```python
from build123d import *

# Parameters (mm, degrees)
F0_R     = 15.875
F1_DEPTH = 5.08
F2_R     = 17.78
F3_DEPTH = 5.08
F4_R     = 9.525
F5_DEPTH = 3.302


with BuildPart() as f1:
    # F0 (on Right) → F1 (new body)
    with BuildSketch(Plane.YZ):
        Circle(F0_R)
        Polygon((0, -14.664697), (-12.7, -7.332348), (-12.7, 7.332348), (0, 14.664697), (12.7, 7.332348), (12.7, -7.332348), align=None, mode=Mode.SUBTRACT)
    extrude(amount=F1_DEPTH)

    # F2 (on face) → F3 (join)
    with BuildSketch(Plane.YZ.offset(5.08)):
        Circle(F2_R)
    extrude(amount=F3_DEPTH)

    # F4 (on face) → F5 (cut)
    with BuildSketch(Plane(origin=(5.08, 0, 0), x_dir=(0, -1, 0), z_dir=(-1, 0, 0))):
        Circle(F4_R)
    extrude(amount=-F5_DEPTH, mode=Mode.SUBTRACT)


solid = f1.part
```
Check sheet for the modelled part. Datum: model origin and axes. Units: mm. A direction names the side the tool comes from. Coordinates: 2 decimals unless noted, no trailing zeros. Write each loop counter-clockwise with the first axis right and the second up, starting at its lowest first coordinate (ties: lowest second). Pieces come first, ordered by that corner, then holes. Notation, with made-up numbers: M 10.25,73.5 L 53.25,73.5 A25 ccw 53.25,104.5 Z; hole C 50,10.25 d3. An arc over 180 degrees is marked long. Write item = value, one per line. Start each with the question number.
1. Sectioned sample at B-B (z = 0). Record the cut outline in (x, y) (3 decimals), then the cut area to 3 significant figures.
2. Thickness scan on probe 1 along Z at (x, y) = (6.65, 0) (3 decimals); probe 2 along X at (y, z) = (-5, 2.5); probe 3 along X at (y, z) = (8, 8). Record the ranges inside material, lowest first.
3. Go/stop test with flat-tipped pins: pin 1 (1.5 mm diameter, centred on x = 1.5, z = -2, fed in from +Y); pin 2 (15 mm diameter, centred on y = 3.5, z = -3.5, fed in from -X); pin 3 (2.5 mm diameter, centred on x = 2.5, z = -2, fed in from -Y). Record where each tip stops, or that it passes through.
4. Sectioned sample at C-C (y = -11). Record the cut outline in (x, z).
5. Sectioned sample at A-A (x = 4.5). Record the cut outline in (y, z) (3 decimals).
6. Mould release check, pull along Y, two halves, no side actions. Record for faces 1 (the cylindrical face through (6.708, 7.559, -5.796)), 2 (the flat face through (8.382, 0, 0)), 3 (the cylindrical face through (7.58, -3.85, -17.36)), 4 (the flat face through (0, 7, 11)): pulls with the +Y half, pulls with the -Y half, needs draft (parallel to the pull), parting line crosses it, or undercut.
7. Sectioned sample at D-D (y = -4.5). Record the cut outline in (x, z).
8. Tool access check on faces 5 (the flat face through (3, 12.7, 0)), 6 (the flat face through (10.16, 0, 0)). Record the directions out of +Z, -Z, +X, -X, +Y, -Y that give a thin tool (end or side, any length) a straight path to the whole face; none if there is none.
The answers:
q1.outline = M 0,-15.875 L 5.08,-15.875 L 5.08,-17.78 L 10.16,-17.78 L 10.16,17.78 L 5.08,17.78 L 5.08,15.875 L 0,15.875 L 0,12.7 L 5.08,12.7 L 5.08,9.525 L 8.382,9.525 L 8.382,-9.525 L 5.08,-9.525 L 5.08,-12.7 L 0,-12.7 Z
q1.area = 150 mm²
q2.probe_1 = -17.78 to -9.525, 9.525 to 17.78
q2.probe_2 = 8.38 to 10.16
q2.probe_3 = 5.08 to 10.16
q3.pin_1 = 15.83
q3.pin_2 = 5.08
q3.pin_3 = -15.86
q4.outline = M 0,-11.45 L 5.08,-11.45 L 5.08,-13.97 L 10.16,-13.97 L 10.16,13.97 L 5.08,13.97 L 5.08,11.45 L 0,11.45 L 0,8.31 L 5.08,8.31 L 5.08,-8.31 L 0,-8.31 Z
q5.outline = C 0,0 d31.75; hole M -12.7,-7.332 L 0,-14.665 L 12.7,-7.332 L 12.7,7.332 L 0,14.665 L -12.7,7.332 Z
q6.face_1 = undercut
q6.face_2 = undercut
q6.face_3 = parting line crosses it
q6.face_4 = needs draft
q7.outline = M 0,-15.22 L 5.08,-15.22 L 5.08,-17.2 L 10.16,-17.2 L 10.16,17.2 L 5.08,17.2 L 5.08,15.22 L 0,15.22 L 0,12.07 L 5.08,12.07 L 5.08,8.39 L 8.38,8.39 L 8.38,-8.39 L 5.08,-8.39 L 5.08,-12.07 L 0,-12.07 Z
q8.face_5 = -X
q8.face_6 = +Z, -Z, +X, +Y, -Y
